Can you work these out from the model? Positions are in its coordinate system, mm. A direction names the side the tool comes from. Round coordinates to 2 decimals unless told otherwise and drop trailing zeros. Write each loop counter-clockwise with the first axis right and the second up, starting at its lowest first coordinate (ties: lowest second). Pieces come first, ordered by that corner, then holes.
Q1. If we section it at B-B (x = 0): Please give me the cut outline in (y, z), plus the area to 3 significant figures.
Q2. For faces 1 (the flat face through (-15.81, 0.61, -1.26)), 2 (the flat face through (21.8, 4, 0)), 3 (the flat face through (18.909, 5.144, 8.956)), 4 (the flat face through (-25, 4, 10)), which set-ups out of +Z, -Z, +X, -X, +Y, -Y let a thin tool reach every point of the face, with its end or its side?
Q3. If we section it at A-A (x = -7): Please give me the cut outline in (y, z), plus the area to 3 significant figures.
Q4. If we section it at C-C (x = 26): Please give me the cut outline in (y, z).
Q5. Please list where these lines run through material, in increasing order: line 1 along Z through (x, y) = (26, 6); line 2 along X through (y, z) = (2.5, -8); line 3 along Z through (x, y) = (24.05, 6.2).
Q6. I'm going to push flat-ended pins straight in: pin 1 Ø1 at (x, y) = (19, 5.5) entering from -Z; pin 2 Ø1.5 at (y, z) = (8, -5.5) entering from -X; pin 3 Ø1.5 at (x, y) = (-25.5, 3) entering from +Z; pin 4 Ø3.5 at (y, z) = (6.2, 0) entering from +X. Where does each tip first touch, or does it pass through?
Q7. If we section it at D-D (z = -16.5): Please give me the cut outline in (x, y), plus the area to 3 significant figures.
Q8. We'd pull the mould along Y, two halves only. Please class faces 5 (the flat face through (25, 11.2, 0)), 6 (the flat face through (26.828, 9.559, -1.976)), 7 (the flat face through (-28.8, 2.8, 2.4)), 8 (the flat face through (27, 6, -3.897)): +Y half, -Y half, draft (parallel to the pull), parting line (faces both ways), or undercut.
from build123d import *

# Parameters (mm, degrees)
ESBO_O1_W                = 60
ESBO_O1_H                = 55
RESSALTO_EXTRUS_O1_DEPTH = 1.2
ESBO_O2_W                = 22
ESBO_O2_H                = 21.5
CORTE_EXTRUS_O1_DEPTH    = 41.714739346
RESSALTO_EXTRUS_O2_DEPTH = 8
ESBO_O4_R                = 1.5
CORTE_EXTRUS_O2_DEPTH    = 7
ESBO_O5_R                = 1.5
CORTE_EXTRUS_O3_DEPTH    = 7
ESBO_O6_R                = 1.5
CORTE_EXTRUS_O4_DEPTH    = 7
FILETE1_R                = 3
FILETE2_R                = 3
FILETE3_R                = 3
FILETE4_R                = 3
ESBO_O8_W                = 7
ESBO_O8_H                = 20
RESSALTO_EXTRUS_O3_DEPTH = 10
CORTE_EXTRUS_O6_DEPTH    = 4
ESBO_O11_R               = 2
CORTE_EXTRUS_O7_DEPTH    = 10
CORTE_EXTRUS_O8_DEPTH    = 4
CORTE_EXTRUS_O9_START    = -10
ESBO_O13_R               = 2
CORTE_EXTRUS_O9_DEPTH    = 10
FILETE5_R                = 5
FILETE6_R                = 5
FILETE7_R                = 5
FILETE9_R                = 5


with BuildPart() as part:
    # Esboço1 → Ressalto-extrusão1 (new body)
    with BuildSketch(Plane(origin=(0, 0, 0), x_dir=(1, 0, 0), z_dir=(0, 1, 0))):
        Rectangle(ESBO_O1_W, ESBO_O1_H)
    extrude(amount=RESSALTO_EXTRUS_O1_DEPTH)

    # Esboço2 → Corte-extrusão1 (cut, through all)
    with BuildSketch(Plane(origin=(0, 1.2, 0), x_dir=(1, 0, 0), z_dir=(0, 1, 0))):
        with Locations((0, -4.680960194)):
            Rectangle(ESBO_O2_W, ESBO_O2_H)
        with BuildLine():
            Line((-20.75, -5.680960194), (-11, -15.430960194))
            Line((-11, -15.430960194), (-11, 6.069039806))
            Line((-11, 6.069039806), (-20.75, -3.680960194))
            ThreePointArc((-20.75, -3.680960194), (-21.131966011, -4.680960194), (-20.75, -5.680960194))
        make_face()
        with BuildLine():
            Line((11, 6.069039806), (11, -15.430960194))
            Line((11, -15.430960194), (20.75, -5.680960194))
            ThreePointArc((20.75, -5.680960194), (21.131966011, -4.680960194), (20.75, -3.680960194))
            Line((20.75, -3.680960194), (11, 6.069039806))
        make_face()
    extrude(amount=-CORTE_EXTRUS_O1_DEPTH, mode=Mode.SUBTRACT)

    # Esboço3 → Ressalto-extrusão2 (add)
    with BuildSketch(Plane(origin=(0, 1.2, 0), x_dir=(1, 0, 0), z_dir=(0, 1, 0))):
        Polygon((-10.998427125, -17.430960194), (10.998427125, -17.430960194), (11.828427125, -17.430960194), (19.606601718, -9.652785601), (18.192388155, -8.238572039), (11, -15.430960194), (-11, -15.430960194), (-18.681875297, -7.749084898), (-20.096088859, -9.16329846), (-11.828427125, -17.430960194), align=None)
    extrude(amount=RESSALTO_EXTRUS_O2_DEPTH)

    # Esboço4 → Corte-extrusão2 (cut)
    with BuildSketch(Plane(origin=(13.215480097, 0, 13.215480097), x_dir=(-0.7071067811865465, 0, 0.7071067811865487), z_dir=(-0.7071067811865487, 0, -0.7071067811865465))):
        with Locations((-1.366837999, 4.2)):
            Circle(ESBO_O4_R)
    extrude(amount=-CORTE_EXTRUS_O2_DEPTH, mode=Mode.SUBTRACT)

    # Esboço5 → Corte-extrusão3 (cut)
    with BuildSketch(Plane(origin=(0, 0, 15.430960194), x_dir=(-1, 0, 0), z_dir=(0, 0, -1))):
        with Locations((0, 4.2)):
            Circle(ESBO_O5_R)
    extrude(amount=-CORTE_EXTRUS_O3_DEPTH, mode=Mode.SUBTRACT)

    # Esboço6 → Corte-extrusão4 (cut)
    with BuildSketch(Plane(origin=(-13.215480097, 0, 13.215480097), x_dir=(-0.7071067811865466, 0, -0.7071067811865485), z_dir=(0.7071067811865485, 0, -0.7071067811865466))):
        with Locations((1.366837999, 4.2)):
            Circle(ESBO_O6_R)
    extrude(amount=-CORTE_EXTRUS_O4_DEPTH, mode=Mode.SUBTRACT)

    # Filete1
    filete1_edges = [part.edges().sort_by_distance(p)[0] for p in [
        (-30, 0.6, -27.5),
    ]]
    fillet(filete1_edges, radius=FILETE1_R)

    # Filete2
    filete2_edges = [part.edges().sort_by_distance(p)[0] for p in [
        (30, 0.6, -27.5),
    ]]
    fillet(filete2_edges, radius=FILETE2_R)

    # Filete3
    filete3_edges = [part.edges().sort_by_distance(p)[0] for p in [
        (30, 0.6, 27.5),
    ]]
    fillet(filete3_edges, radius=FILETE3_R)

    # Filete4
    filete4_edges = [part.edges().sort_by_distance(p)[0] for p in [
        (-30, 0.6, 27.5),
    ]]
    fillet(filete4_edges, radius=FILETE4_R)

    # Esboço8 → Ressalto-extrusão3 (add)
    with BuildSketch(Plane(origin=(0, 1.2, 0), x_dir=(1, 0, 0), z_dir=(0, 1, 0))):
        with Locations((-25.3, 0)):
            Rectangle(ESBO_O8_W, ESBO_O8_H)
        with Locations((25.3, 0)):
            Rectangle(ESBO_O8_W, ESBO_O8_H)
    extrude(amount=RESSALTO_EXTRUS_O3_DEPTH)

    # Esboço9 → Corte-extrusão6 (cut)
    with BuildSketch(Plane.ZY.offset(28.8)):
        Polygon((0, 1.7), (3.897114317, 3.95), (3.897114317, 8.45), (0, 10.7), (-3.897114317, 8.45), (-3.897114317, 3.95), align=None)
    extrude(amount=-CORTE_EXTRUS_O6_DEPTH, mode=Mode.SUBTRACT)

    # Esboço11 → Corte-extrusão7 (cut)
    with BuildSketch(Plane.ZY.offset(24.8)):
        with Locations((0, 6.2)):
            Circle(ESBO_O11_R)
    extrude(amount=-CORTE_EXTRUS_O7_DEPTH, mode=Mode.SUBTRACT)

    # Esboço12 → Corte-extrusão8 (cut)
    with BuildSketch(Plane(origin=(28.8, 0, 0), x_dir=(0, 0, -1), z_dir=(1, 0, 0))):
        Polygon((0, 1.7), (3.897114317, 3.95), (3.897114317, 8.45), (0, 10.7), (-3.897114317, 8.45), (-3.897114317, 3.95), align=None)
    extrude(amount=-CORTE_EXTRUS_O8_DEPTH, mode=Mode.SUBTRACT)

    # Esboço13 → Corte-extrusão9 (cut)
    with BuildSketch(Plane(origin=(24.8, 0, 0), x_dir=(0, 0, -1), z_dir=(1, 0, 0)).offset(CORTE_EXTRUS_O9_START)):
        with Locations(Location((0, 6.2, 0), (0, 0, 180))):
            Circle(ESBO_O13_R)
    extrude(amount=CORTE_EXTRUS_O9_DEPTH, mode=Mode.SUBTRACT)

    # Filete5
    filete5_edges = [part.edges().sort_by_distance(p)[0] for p in [
        (25.3, 11.2, 10),
    ]]
    fillet(filete5_edges, radius=FILETE5_R)

    # Filete6
    filete6_edges = [part.edges().sort_by_distance(p)[0] for p in [
        (25.3, 11.2, -10),
    ]]
    fillet(filete6_edges, radius=FILETE6_R)

    # Filete7
    filete7_edges = [part.edges().sort_by_distance(p)[0] for p in [
        (-25.3, 11.2, -10),
    ]]
    fillet(filete7_edges, radius=FILETE7_R)

    # Filete9
    filete9_edges = [part.edges().sort_by_distance(p)[0] for p in [
        (-25.3, 11.2, 10),
    ]]
    fillet(filete9_edges, radius=FILETE9_R)


solid = part.part
A:
1. outline: (0, -27.5) - (1.2, -27.5) - (1.2, -6.07) - (0, -6.07) - close; (0, 15.43) - (2.7, 15.43) - (2.7, 17.43) - (1.2, 17.43) - (1.2, 27.5) - (0, 27.5) - close; (5.7, 15.43) - (9.2, 15.43) - (9.2, 17.43) - (5.7, 17.43) - close
1. area: 50.2 mm2
2. face 1: +Y, -Y
2. face 2: +Z, -Z, +Y
2. face 3: -Z, +Y
2. face 4: +Z, -X, +Y
3. outline: (0, -27.5) - (1.2, -27.5) - (1.2, -6.07) - (0, -6.07) - close; (0, 15.43) - (9.2, 15.43) - (9.2, 17.43) - (1.2, 17.43) - (1.2, 27.5) - (0, 27.5) - close
3. area: 56.2 mm2
4. outline: (0, -27.5) - (1.2, -27.5) - (1.2, -10) - (6.2, -10) arc R5 ccw to (11.2, -5) - (11.2, 5) arc R5 ccw to (6.2, 10) - (1.2, 10) - (1.2, 27.5) - (0, 27.5) - close; hole (1.7, 0) - (3.95, -3.9) - (8.45, -3.9) - (10.7, 0) - (8.45, 3.9) - (3.95, 3.9) - close
5. line 1: z = -10 to -3.9, 3.9 to 10
5. line 2: x = -28.8 to -21.8, 21.8 to 28.8
5. line 3: z = -10 to -2, 2 to 10
6. pin 1: stops at z = 8.55
6. pin 2: stops at x = -28.8
6. pin 3: stops at z = 10
6. pin 4: passes through
7. outline: (-30, 0) - (30, 0) - (30, 1.2) - (-30, 1.2) - close
7. area: 72.0 mm2
8. face 5: +Y half
8. face 6: undercut
8. face 7: draft
8. face 8: undercut
